Design review of the part built by this model. Coordinates are the model's own, in mm. Face numbers are marked on the shaded views. A direction names the side the tool comes from. Give positions to 0.01 mm unless a question says otherwise; leave off trailing zeros. Loops run counter-clockwise (first coordinate to the right, second up) from the corner with the lowest first, then second, coordinate; pieces in that order, holes last. Notation, with made-up numbers: (66, 61) - (86, 61) arc R27 ccw to (86, 98) - close; hole circle Ø11 at (88.5, 34.5). An arc over 180 degrees is marked (long way). One line per item, written item: value. Start each with the question number.
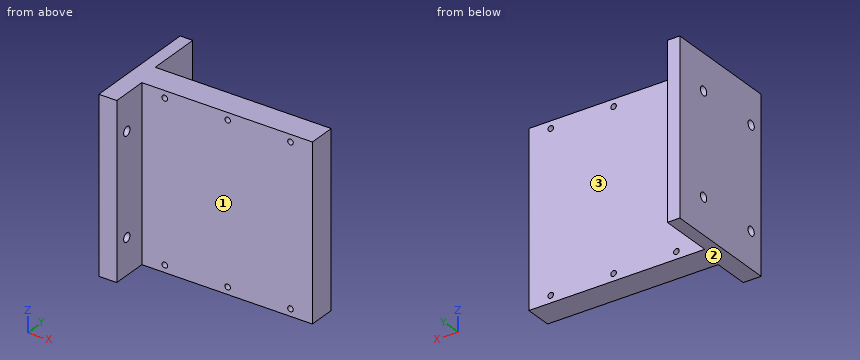
```python
from build123d import *

# Parameters (mm, degrees)
SKIZZE1_W                       = 105
SKIZZE1_H                       = 15
AUFSATZ_LINEAR_AUSTRAGEN1_DEPTH = 96
SKIZZE3_W                       = 7
SKIZZE3_H                       = 96
AUFSATZ_LINEAR_AUSTRAGEN2_DEPTH = 30
SKIZZE4_W                       = 10
SKIZZE4_H                       = 96
AUFSATZ_LINEAR_AUSTRAGEN3_DEPTH = 20
SKIZZE5_R                       = 1.55
SCHNITT_LINEAR_AUSTRAGEN1_DEPTH = 20
SKIZZE6_R                       = 2.5
SCHNITT_LINEAR_AUSTRAGEN2_DEPTH = 20


with BuildPart() as part:
    # Skizze1 → Aufsatz-Linear austragen1 (new body)
    with BuildSketch(Plane.XY):
        Rectangle(SKIZZE1_W, SKIZZE1_H)
    extrude(amount=AUFSATZ_LINEAR_AUSTRAGEN1_DEPTH)

    # Skizze3 → Aufsatz-Linear austragen2 (add)
    with BuildSketch(Plane(origin=(0, 7.5, 0), x_dir=(1, 0, 0), z_dir=(0, 1, 0))):
        with Locations((-49, -48)):
            Rectangle(SKIZZE3_W, SKIZZE3_H)
    extrude(amount=AUFSATZ_LINEAR_AUSTRAGEN2_DEPTH)

    # Skizze4 → Aufsatz-Linear austragen3 (add)
    with BuildSketch(Plane.XZ.offset(7.5)):
        with Locations((-47.5, 48)):
            Rectangle(SKIZZE4_W, SKIZZE4_H)
    extrude(amount=AUFSATZ_LINEAR_AUSTRAGEN3_DEPTH)

    # Skizze5 → Schnitt-Linear austragen1 (cut)
    with BuildSketch(Plane(origin=(0, 7.5, 0), x_dir=(1, 0, 0), z_dir=(0, 1, 0))):
        with Locations(Location((40.3, -92, 0), (0, 0, 270))):
            Circle(SKIZZE5_R)
        with Locations(Location((40.3, -4, 0), (0, 0, 270))):
            Circle(SKIZZE5_R)
        with Locations(Location((5.3, -4, 0), (0, 0, 270))):
            Circle(SKIZZE5_R)
        with Locations(Location((5.3, -92, 0), (0, 0, 270))):
            Circle(SKIZZE5_R)
        with Locations(Location((-29.7, -4, 0), (0, 0, 270))):
            Circle(SKIZZE5_R)
        with Locations(Location((-29.7, -92, 0), (0, 0, 270))):
            Circle(SKIZZE5_R)
    extrude(amount=-SCHNITT_LINEAR_AUSTRAGEN1_DEPTH, mode=Mode.SUBTRACT)

    # Skizze6 → Schnitt-Linear austragen2 (cut)
    with BuildSketch(Plane(origin=(-42.5, 0, 0), x_dir=(0, 0, -1), z_dir=(1, 0, 0))):
        with Locations((-76, -19.5)):
            Circle(SKIZZE6_R)
        with Locations((-20, -19.5)):
            Circle(SKIZZE6_R)
    schnitt_linear_austragen2 = extrude(amount=-SCHNITT_LINEAR_AUSTRAGEN2_DEPTH, mode=Mode.SUBTRACT)

    # Spiegeln1: Schnitt-Linear austragen2 across plane
    add(schnitt_linear_austragen2.mirror(Plane.ZX.offset(-0.5)), mode=Mode.SUBTRACT)


solid = part.part
```
(1) Machinability: for the marked faces 1, 2 and 3, which of the approach directions +Z, -Z, +X, -X, +Y, -Y give a long, thin tool a straight path to every point of the face, cutting with its end or side? Answer none if there is none.
(2) Take a section at A-A on x = 40.3. State the section outline as (y, z) points, and give its area (3 significant figures).
(3) Take a section at C-C on y = 18.5. State the section outline as (x, z) points.
(4) To check wall thickness, follow L1, parallel to X at y = -0.5, z = 92; L2, parallel to Z at x = 5, y = 0; L3, parallel to X at y = 33.5, z = 86. State the ranges of each line that lie inside material, in increasing order. Write a range as from..to.
(5) Take a section at B-B on z = 20. State the section outline as (x, y) points, and give its area (3 significant figures).
(6) For pin 1 Ø4 at (x, z) = (-5.5, 12) entering from -Y; pin 2 Ø4 at (x, z) = (-29.7, 4) entering from +Y; pin 3 Ø24 at (y, z) = (26, 61.5) entering from +X, all flat-tipped, find the tip position at first contact; note any pin that passes through.
(7) Take a section at D-D on z = 4. State the section outline as (x, y) points, and give its area (3 significant figures).
Here are the results:
1. face 1: +Z, -Z, +X, -Y
1. face 2: -Z, +X, -X, +Y, -Y
1. face 3: +Z, -Z, +X, +Y
2. outline: (-7.5, 0) - (7.5, 0) - (7.5, 2.45) - (-7.5, 2.45) - close; (-7.5, 5.55) - (7.5, 5.55) - (7.5, 90.45) - (-7.5, 90.45) - close; (-7.5, 93.55) - (7.5, 93.55) - (7.5, 96) - (-7.5, 96) - close
2. area: 1,350 mm²
3. outline: (-52.5, 0) - (-45.5, 0) - (-45.5, 17.5) - (-52.5, 17.5) - close; (-52.5, 22.5) - (-45.5, 22.5) - (-45.5, 73.5) - (-52.5, 73.5) - close; (-52.5, 78.5) - (-45.5, 78.5) - (-45.5, 96) - (-52.5, 96) - close
4. L1: -52.5..-31.25, -28.15..3.75, 6.85..38.75, 41.85..52.5
4. L2: 0..2.48, 5.52..90.48, 93.52..96
4. L3: -52.5..-45.5
5. outline: (-52.5, -27.5) - (-42.5, -27.5) - (-42.5, -22) - (-52.5, -22) - close; (-52.5, -17) - (-42.5, -17) - (-42.5, -7.5) - (52.5, -7.5) - (52.5, 7.5) - (-45.5, 7.5) - (-45.5, 16) - (-52.5, 16) - close; (-52.5, 21) - (-45.5, 21) - (-45.5, 37.5) - (-52.5, 37.5) - close
5. area: 1,900 mm²
6. pin 1: y = -7.5
6. pin 2: y = 7.5
6. pin 3: x = -45.5
7. outline: (-52.5, -27.5) - (-42.5, -27.5) - (-42.5, -7.5) - (-31.25, -7.5) - (-31.25, 7.5) - (-45.5, 7.5) - (-45.5, 37.5) - (-52.5, 37.5) - close; (-28.15, -7.5) - (3.75, -7.5) - (3.75, 7.5) - (-28.15, 7.5) - close; (6.85, -7.5) - (38.75, -7.5) - (38.75, 7.5) - (6.85, 7.5) - close; (41.85, -7.5) - (52.5, -7.5) - (52.5, 7.5) - (41.85, 7.5) - close
7. area: 1,850 mm²
